```python
from build123d import *

# Parameters (mm, degrees)
SKETCH_R      = 6.2
SKETCH_R_2    = 4.125
PAD_DEPTH     = 15
SKETCH001_R   = 15
SKETCH001_R_2 = 4.15
PAD001_DEPTH  = 4


with BuildPart() as part:
    # Sketch → Pad (new body)
    with BuildSketch(Plane.XY):
        Circle(SKETCH_R)
        Circle(SKETCH_R_2, mode=Mode.SUBTRACT)
    extrude(amount=PAD_DEPTH)

    # Sketch001 (on Face4 of Pad) → Pad001 (join)
    with BuildSketch(Plane.XY.offset(15)):
        Circle(SKETCH001_R)
        Circle(SKETCH001_R_2, mode=Mode.SUBTRACT)
    extrude(amount=PAD001_DEPTH)


solid = part.part
```
Model file for the job. Use its own axes, mm. A direction names the side the tool comes from. Give positions to 0.01 mm unless a question says otherwise; leave off trailing zeros. Write each loop counter-clockwise with the first axis right and the second up, starting at its lowest first coordinate (ties: lowest second). Pieces come first, ordered by that corner, then holes. Notation, with made-up numbers: (20, -2.5) - (68, -2.5) arc R27 ccw to (68, 25.5) - close; hole circle Ø9 at (-2.5, -35.5). An arc over 180 degrees is marked (long way). One line per question, with ' | ' between items. Start each with the question number.
(1) Slice it at A-A on x = 0. Write the cut outline in (y, z) (3 decimals).
(2) Slice it at C-C on z = 10.5. Write the cut outline in (x, y) (3 decimals), plus the area to 3 significant figures.
(3) Pin check, flat tips, straight feed: P1, Ø1, axis at x = 8, y = 6, coming from the -Z side; P2, Ø11, axis at x = 0, y = 0, coming from the -Z side; P3, Ø6.5, axis at x = 0, y = 0, coming from the -Z side; P4, Ø2, axis at x = -4.5, z = 4.5, coming from the -Y side. Stop position of each tip, or through.
(4) Two-plate mould, pull along X, no slides. Class faces 1 (the face through (3.1, -3.1, 19)), 2 (the face through (-14.985, 0.66, 16.972)), 3 (the face through (-0.9, -4.05, 16.97)): +X half, -X half, draft (parallel to the pull), parting line (faces both ways), or undercut.
(5) Slice it at D-D on x = 4.75. Write the cut outline in (y, z).
(6) 3-axis set-ups, long thin cutter, end or side, ignore diameter. For faces 4 (the face through (3.8, -1.6, 7.4)), 5 (the face through (2.86, -5.5, 7.4)): which of +Z, -Z, +X, -X, +Y, -Y reach the whole face in a straight line?
(7) Wall check: line 1 along Y through (x, z) = (0, 7.25) (3 decimals); line 2 along Y through (x, z) = (0, 17.1); line 3 along Z through (x, y) = (-0.25, 13). Give the ranges that are in metal, low to high. Write a range as from..to.
Results below:
1) outline: (-15, 15) - (-6.2, 15) - (-6.2, 0) - (-4.125, 0) - (-4.125, 15) - (-4.15, 15) - (-4.15, 19) - (-15, 19) - close; (4.125, 0) - (6.2, 0) - (6.2, 15) - (15, 15) - (15, 19) - (4.15, 19) - (4.15, 15) - (4.125, 15) - close
2) outline: circle Ø12.4 at (0, 0); hole circle Ø8.25 at (0, 0) | area: 67.3 mm^2
3) P1: z = 15 | P2: z = 0 | P3: through | P4: y = -5.12
4) face 1: draft | face 2: parting line | face 3: undercut
5) outline: (-14.23, 15) - (-3.98, 15) - (-3.98, 0) - (3.98, 0) - (3.98, 15) - (14.23, 15) - (14.23, 19) - (-14.23, 19) - close
6) face 4: +Z, -Z | face 5: -Z
7) line 1: -6.2..-4.125, 4.125..6.2 | line 2: -15..-4.15, 4.15..15 | line 3: 15..19
